```python
from build123d import *

# Parameters (mm, degrees)
SKETCH3_R = 0.4


with BuildPart() as part:
    # Sweep1: sweep along a path in Sketch2
    with BuildLine(Plane.XY) as sweep1_path:
        Line((0, 0), (3, 0))
        Line((3, 0), (3, 3))
        Line((3, 3), (41.05, 3))
        Line((41.05, 3), (41.05, 6))
        Line((41.05, 6), (44.05, 6))
    # Sketch3 → Sweep1 (sweep)
    with BuildSketch(Plane(origin=(0, 0, 0), x_dir=(0, 0, -1), z_dir=(1, 0, 0))):
        Circle(SKETCH3_R)
    sweep(path=sweep1_path.line, transition=Transition.RIGHT)


solid = part.part
```
Input: part model. Units: mm. Frame: model coordinates. Give positions to 0.01 mm unless a question says otherwise; leave off trailing zeros. Order: outer loops, then holes, each group sorted by start corner. A loop starts at its lowest first (then second) coordinate and runs counter-clockwise, first axis right, second up. Notation, with made-up numbers: (-16, 57.25) - (22, 57.25) arc R15 ccw to (22, 82.25) - close; hole circle Ø9 at (56, 28.25). An arc over 180 degrees is marked (long way). Use a Markdown table: item, result.
(1) Line query: line 1 (X direction, y = 0.75, z = -0.05); line 2 (X direction, y = 6.25, z = -0.05). Output: solid intervals per line, ascending. Write a range as from..to.
Computed values:
| item | result |
|---|---|
| line 1 | x = 2.6..3.4 |
| line 2 | x = 40.65..44.05 |
(2) Section query C-C (x = 3). Output: boundary loops of the cut face in (y, z).
Computed values:
| item | result |
|---|---|
| outline | (0, -0.4) - (3, -0.4) arc R0.4 ccw to (3, 0.4) - (0, 0.4) arc R0.4 ccw to start |
(3) Section query D-D (y = 3). Output: boundary loops of the cut face in (x, z).
Computed values:
| item | result |
|---|---|
| outline | (3, -0.4) - (41.05, -0.4) arc R0.4 ccw to (41.05, 0.4) - (3, 0.4) arc R0.4 ccw to start |
(4) Pin query (flat end, axial travel): pin 1 (1.5 mm diameter, centred on x = 28, y = 3.5, fed in from -Z); pin 2 (4 mm diameter, centred on x = 33, y = 0.5, fed in from +Z). Return the tip coordinate at first contact, or that it passes through.
Computed values:
| item | result |
|---|---|
| pin 1 | stops at z = -0.4 |
| pin 2 | passes through |
(5) Section query B-B (y = 5). Output: boundary loops of the cut face in (x, z).
Computed values:
| item | result |
|---|---|
| outline | circle Ø0.8 at (41.05, 0) |
(6) Section query A-A (x = 29). Output: boundary loops of the cut face in (y, z), then the cut area to 3 significant figures.
Computed values:
| item | result |
|---|---|
| outline | circle Ø0.8 at (3, 0) |
| area | 0.503 mm2 |
